Verification items for this drawing (mm, ordinates from the low corner). A direction names the side the tool comes from. Give positions to 0.01 mm unless a question says otherwise; leave off trailing zeros. Write each loop counter-clockwise with the first axis right and the second up, starting at its lowest first coordinate (ties: lowest second). Pieces come first, ordered by that corner, then holes. Notation, with made-up numbers: (27.25, 34) -> (72.25, 34) arc R20 ccw to (72.25, 70) -> close; hole circle Ø5 at (58, 52). An arc over 180 degrees is marked (long way). One line per item, written item: value.
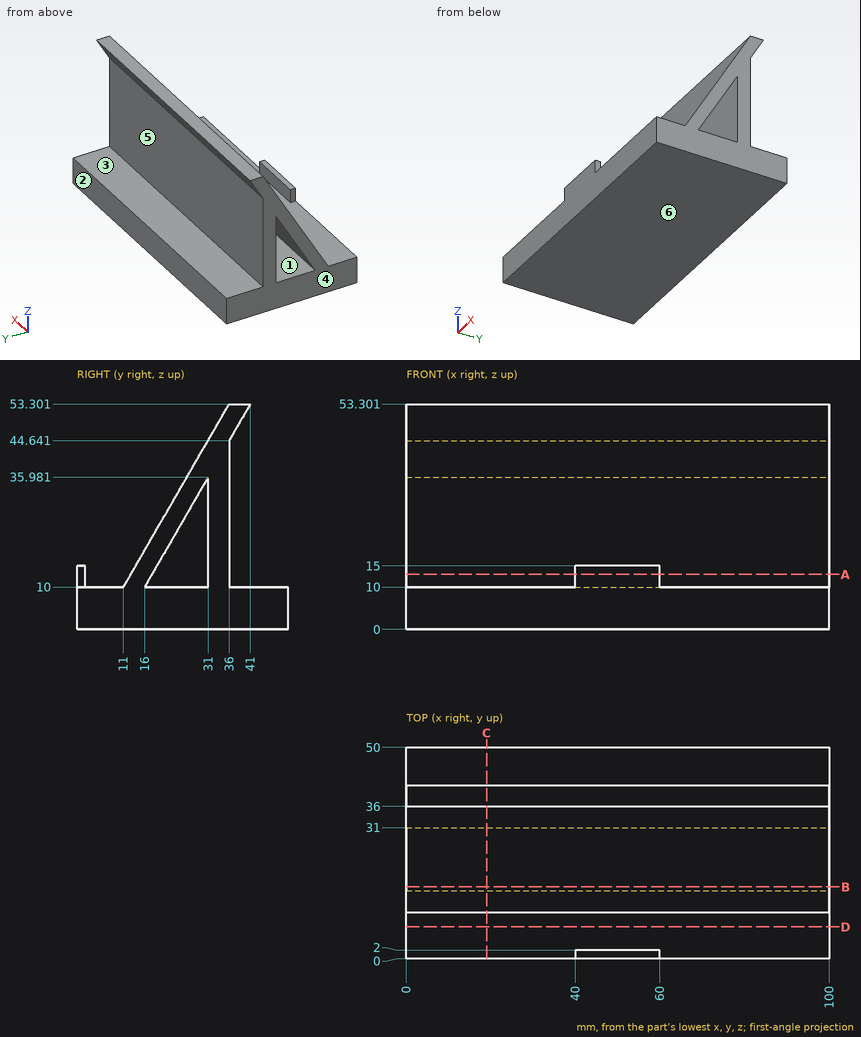
1) Sectioned sample at C-C on x = 19. Record the cut outline in (y, z).
Verdict:
outline: (0, 0) -> (50, 0) -> (50, 10) -> (36, 10) -> (36, 44.64) -> (41, 53.3) -> (36, 53.3) -> (11, 10) -> (0, 10) -> close; hole (16, 10) -> (31, 10) -> (31, 35.98) -> close
2) Mould release check, pull along Z, two halves, no side actions. Record for the marked faces 4, 5 and 6: released by +Z, released by -Z, zero draft, split by the parting line, or undercut.
Verdict:
face 4: zero draft
face 5: undercut
face 6: released by -Z
3) Tool access check on the marked faces 1, 2 and 3. Record the directions out of +Z, -Z, +X, -X, +Y, -Y that give a thin tool (end or side, any length) a straight path to the whole face; none if there is none.
Verdict:
face 1: +X, -X
face 2: +Z, -Z, +X, -X, +Y
face 3: +X, -X, +Y
4) Sectioned sample at A-A on z = 13. Record the cut outline in (x, y).
Verdict:
outline: (0, 12.73) -> (100, 12.73) -> (100, 17.73) -> (0, 17.73) -> close; (0, 31) -> (100, 31) -> (100, 36) -> (0, 36) -> close; (40, 0) -> (60, 0) -> (60, 2) -> (40, 2) -> close
5) Scan lines: probe 1 along Z at (x, y) = (90, 18) (1 decimal); probe 2 along Z at (x, y) = (91.5, 21); probe 3 along Y at (x, z) = (69.5, 14). Record each from-to range of solid material in increasing order.
Verdict:
probe 1: 0 to 10, 13.5 to 22.1
probe 2: 0 to 10, 18.66 to 27.32
probe 3: 13.31 to 18.31, 31 to 36
6) Sectioned sample at B-B on y = 17. Record the cut outline in (x, z), plus the area to 3 significant figures.
Verdict:
outline: (0, 0) -> (100, 0) -> (100, 10) -> (0, 10) -> close; (0, 11.73) -> (100, 11.73) -> (100, 20.39) -> (0, 20.39) -> close
area: 1,870 mm^2
7) Sectioned sample at D-D on y = 7.5. Record the cut outline in (x, z).
Verdict:
outline: (0, 0) -> (100, 0) -> (100, 10) -> (0, 10) -> close
8) Depth check by flat-ended pin: pin 1 Ø9 at (x, y) = (44.5, 3.5) entering from +Z; pin 2 Ø6 at (y, z) = (40, 28) entering from -X; pin 3 Ø16.5 at (x, y) = (36, 20.5) entering from +Z (1 decimal); pin 4 Ø8 at (x, z) = (42.5, 27.5) entering from -Y (1 decimal). Enter the tip coordinate at first touch or a pass-through.
Verdict:
pin 1: z = 15
pin 2: through
pin 3: z = 40.7
pin 4: y = 18.8
